Answer from the drawing. Dimensions are ordinates in mm from the lowest x, y and z of the part. Coordinates: 2 decimals unless noted, no trailing zeros. Loops run counter-clockwise (first coordinate to the right, second up) from the corner with the lowest first, then second, coordinate; pieces in that order, holes last.
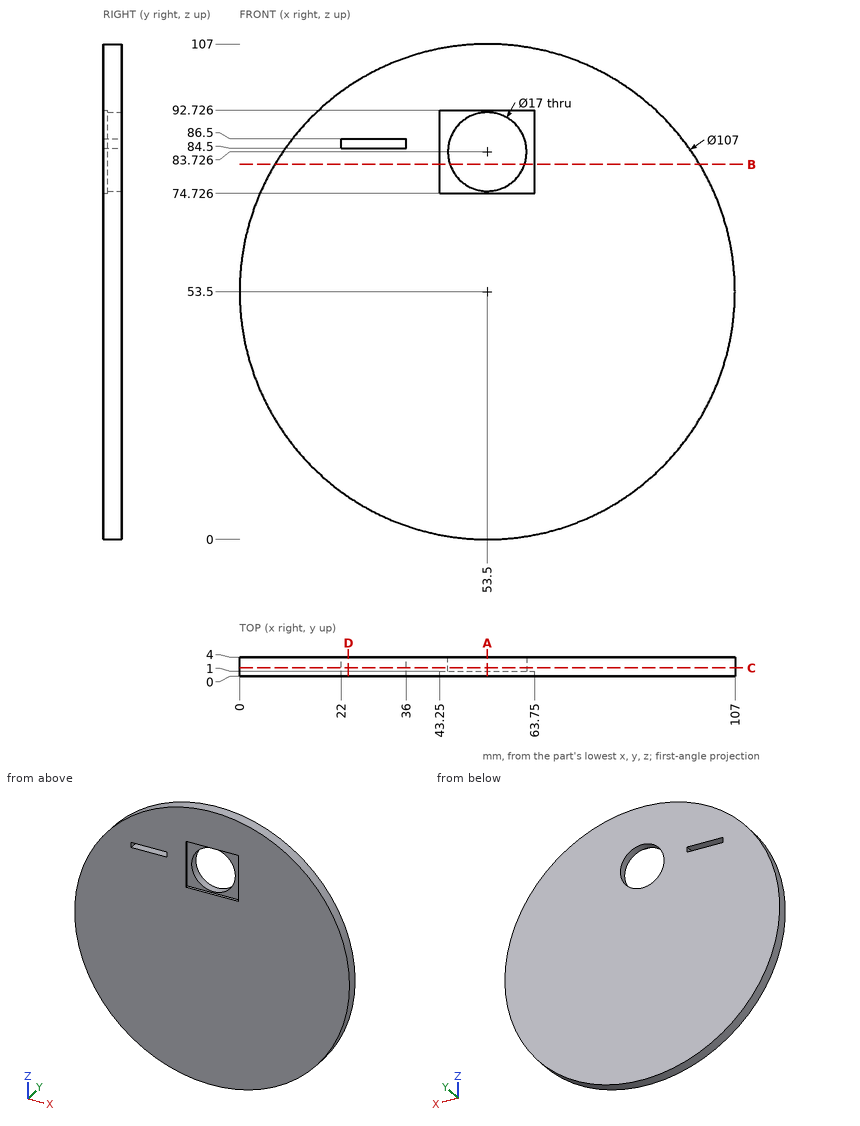
Item 1: A cutting plane is placed at D-D on x = 23.5. Determine the outline of the cut face in (y, z).
Numbers:
outline: (0, 9.2) - (4, 9.2) - (4, 84.5) - (0, 84.5) - close; (0, 86.5) - (4, 86.5) - (4, 97.8) - (0, 97.8) - close
Item 2: A cutting plane is placed at B-B on z = 81. Determine the outline of the cut face in (x, y).
Numbers:
outline: (7.61, 0) - (43.25, 0) - (43.25, 1) - (45.45, 1) - (45.45, 4) - (7.61, 4) - close; (61.55, 1) - (63.75, 1) - (63.75, 0) - (99.39, 0) - (99.39, 4) - (61.55, 4) - close
Item 3: A cutting plane is placed at A-A on x = 53.5. Determine the outline of the cut face in (y, z), then the cut area to 3 significant figures.
Numbers:
outline: (0, 0) - (4, 0) - (4, 75.23) - (1, 75.23) - (1, 74.73) - (0, 74.73) - close; (0, 92.73) - (1, 92.73) - (1, 92.23) - (4, 92.23) - (4, 107) - (0, 107) - close
area: 359 mm2
Item 4: A cutting plane is placed at C-C on y = 1.75. Determine the outline of the cut face in (x, z), then the cut area to 3 significant figures.
Numbers:
outline: circle Ø107 at (53.5, 53.5); hole (22, 84.5) - (36, 84.5) - (36, 86.5) - (22, 86.5) - close; hole circle Ø17 at (53.5, 83.73)
area: 8,740 mm2
Item 5: Given pin 1 (2 mm diameter, centred on x = 32, y = 3, fed in from +Z); pin 2 (10 mm diameter, centred on x = 53.5, z = 83.73, fed in from -Y); pin 3 (0.5 mm diameter, centred on y = 0.5, z = 85, fed in from -X) (1 decimal); pin 4 (1.1 mm diameter, centred on x = 55.5, y = 0.5, fed in from -Z), each flat-ended and moving along its own axis, determine where each tip first touches the part or whether it passes through.
Numbers:
pin 1: stops at z = 102.92
pin 2: passes through
pin 3: stops at x = 10.1
pin 4: stops at z = 0.02
Item 6: Find the intervals of material crossed by line 1 along Z through (x, y) = (53.5, 2.6); line 2 along X through (y, z) = (1.75, 54); line 3 along Z through (x, y) = (32, 0.4), in increasing order.
Numbers:
line 1: z = 0 to 75.23, 92.23 to 107
line 2: x = 0 to 107
line 3: z = 4.51 to 84.5, 86.5 to 102.49
